The listing builds one solid part. Answer for the finished solid, in the listing's coordinates (mm). A direction names the side the tool comes from. Give positions to 0.01 mm unless a question says otherwise; leave off trailing zeros. Loops run counter-clockwise (first coordinate to the right, second up) from the corner with the lowest first, then second, coordinate; pieces in that order, holes last.
Item 1: The mould has two halves that part along X. Classify faces 4 (the face through (61.99, 22.85, 1.01)), 5 (the face through (127, 115, -1)), 6 (the face through (23.01, 42.15, 1.01)), 7 (the face through (168, 1, -5)): pulls with the +X half, pulls with the -X half, needs draft (parallel to the pull), parting line crosses it, or undercut.
Item 2: Section C-C, the plane z = -5.5 is taken. Give the vertices of the cut face in (x, y).
Item 3: Section B-B, the plane y = 79.5 is taken. Give the vertices of the cut face in (x, z).
Item 4: Section A-A, the plane x = 95 is taken. Give the vertices of the cut face in (y, z), and give its area (3 significant figures).
Item 5: This flat-tipped pin is pushed along its axis until it touches: pin 1 Ø10 at (x, y) = (136.5, 73.5) entering from -Z. Where does it stop, or does it pass through?
Item 6: A tool of negligible diameter and unlimited length cuts with its end or side. For faces 1 (the face through (168, 59, -6)), 2 (the face through (121.416, 27.297, 0.986)), 3 (the face through (62.15, 41.99, 1.01)), from which of +Z, -Z, +X, -X, +Y, -Y can it reach the whole face along a straight path? Write none if from no direction.
Item 7: Section D-D, the plane x = 144 is taken. Give the vertices of the cut face in (y, z), and give its area (3 significant figures).
Item 8: Consider line 1 along Y through (x, z) = (26.5, -0.3); line 2 along Y through (x, z) = (145.5, -7.5); line 3 along Y through (x, z) = (46.5, 0.7). Determine where each line is inside the solid, lowest interval first.
from build123d import *

# Parameters (mm, degrees)
SKETCH1_W               = 170
SKETCH1_H               = 120
BOSS_EXTRUDE1_DEPTH     = 10
SHELL1_T                = -2
FILLET1_R               = 5
SKETCH2_R               = 7
CUT_EXTRUDE1_DEPTH      = 209.32666656
SKETCH3_R               = 9
BOSS_EXTRUDE2_DEPTH     = 2
SKETCH4_W               = 70
SKETCH4_H               = 25
CUT_EXTRUDE2_DEPTH      = 209.32666656
SKETCH10_W              = 45
SKETCH10_H              = 25
BOSS_EXTRUDE4_DEPTH     = 2
FILL_START              = -2
FILL_PATTERN2_OUTLINE_R = 1.5
FILL_PATTERN2_DEPTH     = 4
FILLET2_R               = 10
SKETCH11_W              = 84
SKETCH11_H              = 15
CUT_EXTRUDE3_DEPTH      = 209.32666656


# Read off the part's stored shape, not the designer's step: Fill Pattern2
with BuildPart() as part:
    # Sketch1 → Boss-Extrude1 (new body)
    with BuildSketch(Plane.XY):
        with Locations((85, 60)):
            Rectangle(SKETCH1_W, SKETCH1_H)
    extrude(amount=-BOSS_EXTRUDE1_DEPTH)

    # Shell1
    shell1_openings = [part.faces().sort_by_distance(p)[0] for p in [
        (85, 60, -10),
    ]]
    offset(amount=SHELL1_T, openings=shell1_openings, kind=Kind.INTERSECTION)

    # Fillet1
    fillet1_edges = [part.edges().sort_by_distance(p)[0] for p in [
        (2, 2, -6),
        (2, 118, -6),
        (168, 118, -6),
        (168, 2, -6),
        (0, 120, -5),
        (170, 120, -5),
        (170, 0, -5),
        (0, 0, -5),
    ]]
    fillet(fillet1_edges, radius=FILLET1_R)

    # Sketch2 → Cut-Extrude1 (cut, through all)
    with BuildSketch(Plane.XY):
        with Locations((130, 30)):
            Circle(SKETCH2_R)
    extrude(amount=-CUT_EXTRUDE1_DEPTH, mode=Mode.SUBTRACT)

    # Sketch3 → Boss-Extrude2 (add)
    with BuildSketch(Plane.XY):
        with Locations(Location((130, 30, 0), (0, 0, 180))):
            Circle(SKETCH3_R)
    extrude(amount=BOSS_EXTRUDE2_DEPTH)

    # Sketch4 → Cut-Extrude2 (cut, through all)
    with BuildSketch(Plane.XY):
        with Locations((85, 77.5)):
            Rectangle(SKETCH4_W, SKETCH4_H)
    extrude(amount=-CUT_EXTRUDE2_DEPTH, mode=Mode.SUBTRACT)

    # Sketch10 → Boss-Extrude4 (add)
    with BuildSketch(Plane.XY):
        with Locations((42.5, 32.5)):
            Rectangle(SKETCH10_W, SKETCH10_H)
    extrude(amount=BOSS_EXTRUDE4_DEPTH)

    # Fill Pattern2 outline → Fill Pattern2 (cut)
    with BuildSketch(Plane.XY.offset(FILL_START)):
        with Locations((42.5, 32.5)):
            Circle(FILL_PATTERN2_OUTLINE_R)
        with Locations((30.5, 32.5)):
            Circle(FILL_PATTERN2_OUTLINE_R)
        with Locations((30.5, 36.5)):
            Circle(FILL_PATTERN2_OUTLINE_R)
        with Locations((30.5, 40.5)):
            Circle(FILL_PATTERN2_OUTLINE_R)
        with Locations((26.5, 24.5)):
            Circle(FILL_PATTERN2_OUTLINE_R)
        with Locations((30.5, 24.5)):
            Circle(FILL_PATTERN2_OUTLINE_R)
        with Locations((42.5, 40.5)):
            Circle(FILL_PATTERN2_OUTLINE_R)
        with Locations((30.5, 28.5)):
            Circle(FILL_PATTERN2_OUTLINE_R)
        with Locations((46.5, 40.5)):
            Circle(FILL_PATTERN2_OUTLINE_R)
        with Locations((26.5, 28.5)):
            Circle(FILL_PATTERN2_OUTLINE_R)
        with Locations((26.5, 32.5)):
            Circle(FILL_PATTERN2_OUTLINE_R)
        with Locations((26.5, 36.5)):
            Circle(FILL_PATTERN2_OUTLINE_R)
        with Locations((26.5, 40.5)):
            Circle(FILL_PATTERN2_OUTLINE_R)
        with Locations((54.5, 32.5)):
            Circle(FILL_PATTERN2_OUTLINE_R)
        with Locations((50.5, 28.5)):
            Circle(FILL_PATTERN2_OUTLINE_R)
        with Locations((42.5, 28.5)):
            Circle(FILL_PATTERN2_OUTLINE_R)
        with Locations((58.5, 40.5)):
            Circle(FILL_PATTERN2_OUTLINE_R)
        with Locations((54.5, 28.5)):
            Circle(FILL_PATTERN2_OUTLINE_R)
        with Locations((50.5, 24.5)):
            Circle(FILL_PATTERN2_OUTLINE_R)
        with Locations((38.5, 28.5)):
            Circle(FILL_PATTERN2_OUTLINE_R)
        with Locations((58.5, 36.5)):
            Circle(FILL_PATTERN2_OUTLINE_R)
        with Locations((50.5, 36.5)):
            Circle(FILL_PATTERN2_OUTLINE_R)
        with Locations((46.5, 32.5)):
            Circle(FILL_PATTERN2_OUTLINE_R)
        with Locations((50.5, 40.5)):
            Circle(FILL_PATTERN2_OUTLINE_R)
        with Locations((46.5, 36.5)):
            Circle(FILL_PATTERN2_OUTLINE_R)
        with Locations((54.5, 36.5)):
            Circle(FILL_PATTERN2_OUTLINE_R)
        with Locations((50.5, 32.5)):
            Circle(FILL_PATTERN2_OUTLINE_R)
        with Locations((46.5, 28.5)):
            Circle(FILL_PATTERN2_OUTLINE_R)
        with Locations((54.5, 40.5)):
            Circle(FILL_PATTERN2_OUTLINE_R)
        with Locations((42.5, 36.5)):
            Circle(FILL_PATTERN2_OUTLINE_R)
        with Locations((38.5, 24.5)):
            Circle(FILL_PATTERN2_OUTLINE_R)
        with Locations((34.5, 24.5)):
            Circle(FILL_PATTERN2_OUTLINE_R)
        with Locations((34.5, 28.5)):
            Circle(FILL_PATTERN2_OUTLINE_R)
        with Locations((34.5, 32.5)):
            Circle(FILL_PATTERN2_OUTLINE_R)
        with Locations((34.5, 36.5)):
            Circle(FILL_PATTERN2_OUTLINE_R)
        with Locations((34.5, 40.5)):
            Circle(FILL_PATTERN2_OUTLINE_R)
        with Locations((38.5, 40.5)):
            Circle(FILL_PATTERN2_OUTLINE_R)
        with Locations((58.5, 32.5)):
            Circle(FILL_PATTERN2_OUTLINE_R)
        with Locations((38.5, 32.5)):
            Circle(FILL_PATTERN2_OUTLINE_R)
        with Locations((46.5, 24.5)):
            Circle(FILL_PATTERN2_OUTLINE_R)
        with Locations((54.5, 24.5)):
            Circle(FILL_PATTERN2_OUTLINE_R)
        with Locations((58.5, 28.5)):
            Circle(FILL_PATTERN2_OUTLINE_R)
        with Locations((38.5, 36.5)):
            Circle(FILL_PATTERN2_OUTLINE_R)
        with Locations((42.5, 24.5)):
            Circle(FILL_PATTERN2_OUTLINE_R)
        with Locations((58.5, 24.5)):
            Circle(FILL_PATTERN2_OUTLINE_R)
    extrude(amount=FILL_PATTERN2_DEPTH, mode=Mode.SUBTRACT)

    # Fillet2
    fillet2_edges = [part.edges().sort_by_distance(p)[0] for p in [
        (20, 45, 1),
        (20, 20, 1),
        (65, 20, 1),
        (65, 45, 1),
    ]]
    fillet(fillet2_edges, radius=FILLET2_R)

    # Sketch11 → Cut-Extrude3 (cut, through all)
    with BuildSketch(Plane.XY):
        with Locations((85, 112.5)):
            Rectangle(SKETCH11_W, SKETCH11_H)
    extrude(amount=-CUT_EXTRUDE3_DEPTH, mode=Mode.SUBTRACT)


solid = part.part
Worked answers:
1. face 4: undercut
1. face 5: undercut
1. face 6: pulls with the -X half
1. face 7: pulls with the +X half
2. outline: (0, 5) arc R5 ccw to (5, 0) - (165, 0) arc R5 ccw to (170, 5) - (170, 115) arc R5 ccw to (165, 120) - (127, 120) - (127, 118) - (163, 118) arc R5 cw to (168, 113) - (168, 7) arc R5 cw to (163, 2) - (7, 2) arc R5 cw to (2, 7) - (2, 113) arc R5 cw to (7, 118) - (43, 118) - (43, 120) - (5, 120) arc R5 ccw to (0, 115) - close
3. outline: (0, -10) - (2, -10) - (2, -2) - (50, -2) - (50, 0) - (0, 0) - close; (120, -2) - (168, -2) - (168, -10) - (170, -10) - (170, 0) - (120, 0) - close
4. outline: (0, -10) - (2, -10) - (2, -2) - (65, -2) - (65, 0) - (0, 0) - close; (90, -2) - (105, -2) - (105, 0) - (90, 0) - close
4. area: 176 mm2
5. pin 1: stops at z = -2
6. face 1: -Z
6. face 2: +Z
6. face 3: +Z, +Y
7. outline: (0, -10) - (2, -10) - (2, -2) - (118, -2) - (118, -10) - (120, -10) - (120, 0) - (0, 0) - close
7. area: 272 mm2
8. line 1: y = 0 to 23, 26 to 27, 30 to 31, 34 to 35, 38 to 39, 42 to 120
8. line 2: y = 0 to 2, 118 to 120
8. line 3: y = 20 to 23, 26 to 27, 30 to 31, 34 to 35, 38 to 39, 42 to 45
